Verification items for this drawing (mm, ordinates from the low corner). A direction names the side the tool comes from. Coordinates: 2 decimals unless noted, no trailing zeros. Order: outer loops, then holes, each group sorted by start corner. A loop starts at its lowest first (then second) coordinate and runs counter-clockwise, first axis right, second up.
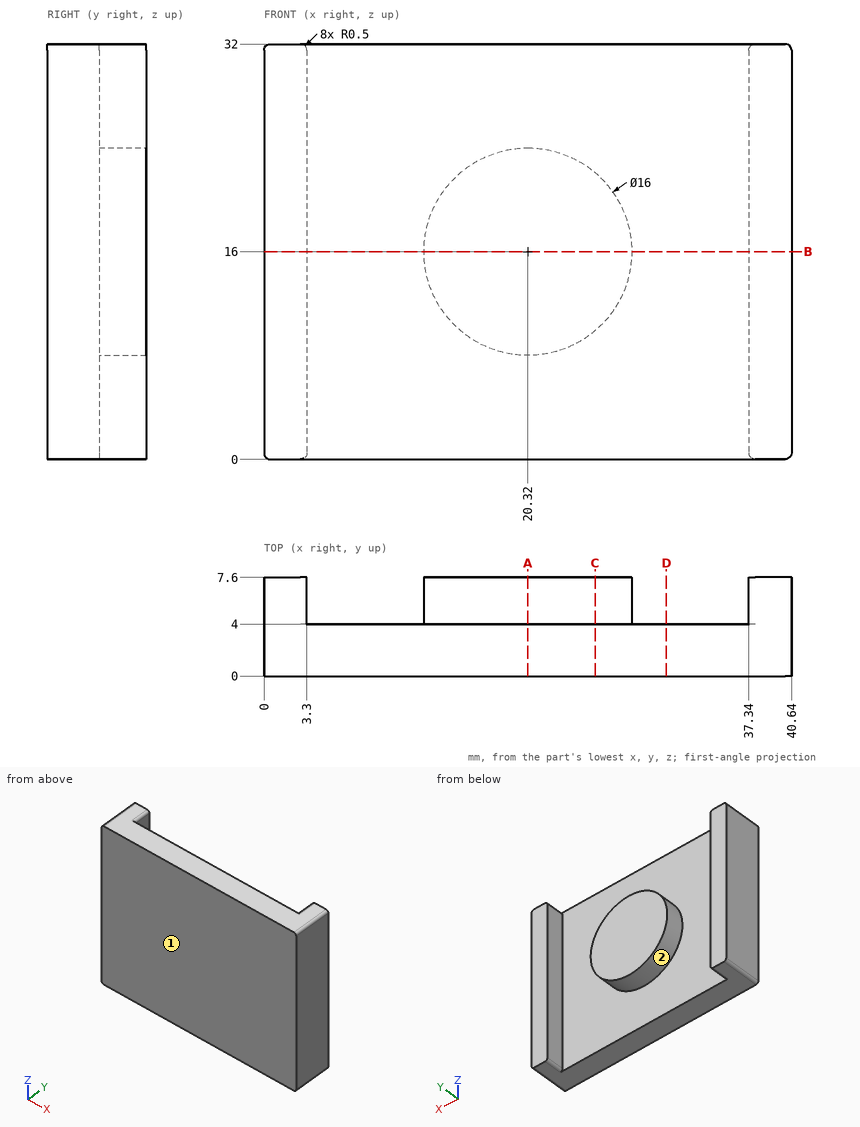
(1) Cross-section at A-A (x = 20.32). Enter the section's corners in (y, z).
Filled in:
outline: (0, 0) - (4, 0) - (4, 8) - (7.6, 8) - (7.6, 24) - (4, 24) - (4, 32) - (0, 32) - close
(2) Tool access check on the marked faces 1 and 2. Record the directions out of +Z, -Z, +X, -X, +Y, -Y that give a thin tool (end or side, any length) a straight path to the whole face; none if there is none.
Filled in:
face 1: +Z, -Z, +X, -X, -Y
face 2: +Y
(3) Cross-section at B-B (z = 16). Enter the section's corners in (x, y).
Filled in:
outline: (0, 0) - (40.64, 0) - (40.64, 7.6) - (37.34, 7.6) - (37.34, 4) - (28.32, 4) - (28.32, 7.6) - (12.32, 7.6) - (12.32, 4) - (3.3, 4) - (3.3, 7.6) - (0, 7.6) - close
(4) Cross-section at C-C (x = 25.5). Enter the section's corners in (y, z), and give its area (3 significant figures).
Filled in:
outline: (0, 0) - (4, 0) - (4, 9.9) - (7.6, 9.9) - (7.6, 22.1) - (4, 22.1) - (4, 32) - (0, 32) - close
area: 172 mm2
(5) Go/stop test with a flat-tipped pin: P1, Ø1.5, axis at x = 23, y = 6.5, coming from the -Z side. Record where the tip stops, or that it passes through.
Filled in:
P1: stops at z = 8.24
(6) Cross-section at D-D (x = 31). Enter the section's corners in (y, z).
Filled in:
outline: (0, 0) - (4, 0) - (4, 32) - (0, 32) - close
(7) Thickness scan on probe 1 along X at (y, z) = (5.5, 16); probe 2 along X at (y, z) = (5.25, 9.5); probe 3 along Y at (x, z) = (20.5, 6). Record the ranges inside material, lowest first.
Filled in:
probe 1: x = 0 to 3.3, 12.32 to 28.32, 37.34 to 40.64
probe 2: x = 0 to 3.3, 15.66 to 24.98, 37.34 to 40.64
probe 3: y = 0 to 4
